```python
from build123d import *

# Parameters (mm, degrees)
CROQUIS2_R              = 0.75
SALIENTE_EXTRUIR1_DEPTH = 2


with BuildPart() as part:
    # Croquis2 → Saliente-Extruir1 (new body)
    with BuildSketch(Plane.XY):
        with BuildLine():
            Line((18.568483774, -2.752576707), (21.714285714, -1.14e-07))
            Line((21.714285714, -1.14e-07), (18.568483781, 2.752576682))
            ThreePointArc((18.568483781, 2.752576682), (18.261705841, 2.936102741), (17.909979159, 3))
            Line((17.909979159, 3), (-17.285714286, 3))
            ThreePointArc((-17.285714286, 3), (-17.992821067, 2.707106781), (-18.285714286, 2))
            Line((-18.285714286, 2), (-18.285714286, -2))
            ThreePointArc((-18.285714286, -2), (-17.992821067, -2.707106781), (-17.285714286, -3))
            Line((-17.285714286, -3), (17.90997918, -3))
            ThreePointArc((17.90997918, -3), (18.261705845, -2.936102747), (18.568483774, -2.752576707))
        make_face()
        with Locations((-16.385714286, 0)):
            Circle(CROQUIS2_R, mode=Mode.SUBTRACT)
        with Locations((-13.985714286, 0)):
            Circle(CROQUIS2_R, mode=Mode.SUBTRACT)
        with Locations((-11.585714286, 0)):
            Circle(CROQUIS2_R, mode=Mode.SUBTRACT)
        with Locations((-9.185714286, 0)):
            Circle(CROQUIS2_R, mode=Mode.SUBTRACT)
        with Locations((-6.785714286, 0)):
            Circle(CROQUIS2_R, mode=Mode.SUBTRACT)
        with Locations((-4.385714286, 0)):
            Circle(CROQUIS2_R, mode=Mode.SUBTRACT)
        with Locations((-1.985714286, 0)):
            Circle(CROQUIS2_R, mode=Mode.SUBTRACT)
        with Locations((0.414285714, 0)):
            Circle(CROQUIS2_R, mode=Mode.SUBTRACT)
        with Locations((2.814285714, 0)):
            Circle(CROQUIS2_R, mode=Mode.SUBTRACT)
        with Locations((5.214285714, 0)):
            Circle(CROQUIS2_R, mode=Mode.SUBTRACT)
        with Locations((7.614285714, 0)):
            Circle(CROQUIS2_R, mode=Mode.SUBTRACT)
        with Locations((10.014285714, 0)):
            Circle(CROQUIS2_R, mode=Mode.SUBTRACT)
        with Locations((12.414285714, 0)):
            Circle(CROQUIS2_R, mode=Mode.SUBTRACT)
        with Locations((14.814285714, 0)):
            Circle(CROQUIS2_R, mode=Mode.SUBTRACT)
    extrude(amount=SALIENTE_EXTRUIR1_DEPTH)


solid = part.part
```
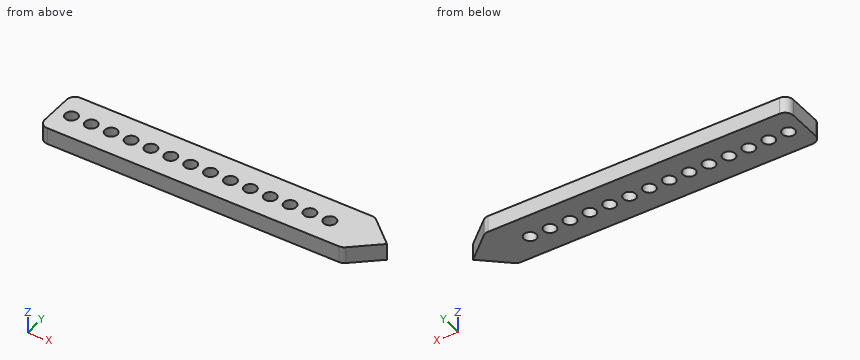
The model under review builds one solid part; all positions refer to its coordinate system, in mm. Round coordinates to 2 decimals unless told otherwise and drop trailing zeros. Loops run counter-clockwise (first coordinate to the right, second up) from the corner with the lowest first, then second, coordinate; pieces in that order, holes last.
1) Consider section B-B on x = 2.5. State the section outline as (y, z) points, then the cut area to 3 significant figures.
Values follow:
outline: (-3, 0) - (-0.68, 0) - (-0.68, 2) - (-3, 2) - close; (0.68, 0) - (3, 0) - (3, 2) - (0.68, 2) - close
area: 9.28 mm2
2) Consider section A-A on z = 1.35. Give the number of separate pieces and of enclosed holes in the cut face, then the cut area to 3 significant figures.
Values follow:
separate pieces: 1
enclosed holes: 14
area: 205 mm2
3) Clearance check with a flat-ended pin moving along its axis: P1, Ø1.4, axis at x = -13.99, y = 0, coming from the -Z side. State where the tip first meets the part, or that it passes through.
Values follow:
P1: passes through
4) Wall thickness on line 1 along Y through (x, z) = (7.5, 1.65); line 2 along Y through (x, z) = (0, 1.8); line 3 along Y through (x, z) = (18, 0.1): over which ranges is each line inside the solid? List them lowest first.
Values follow:
line 1: y = -3 to -0.74, 0.74 to 3
line 2: y = -3 to -0.63, 0.63 to 3
line 3: y = -3 to 3
